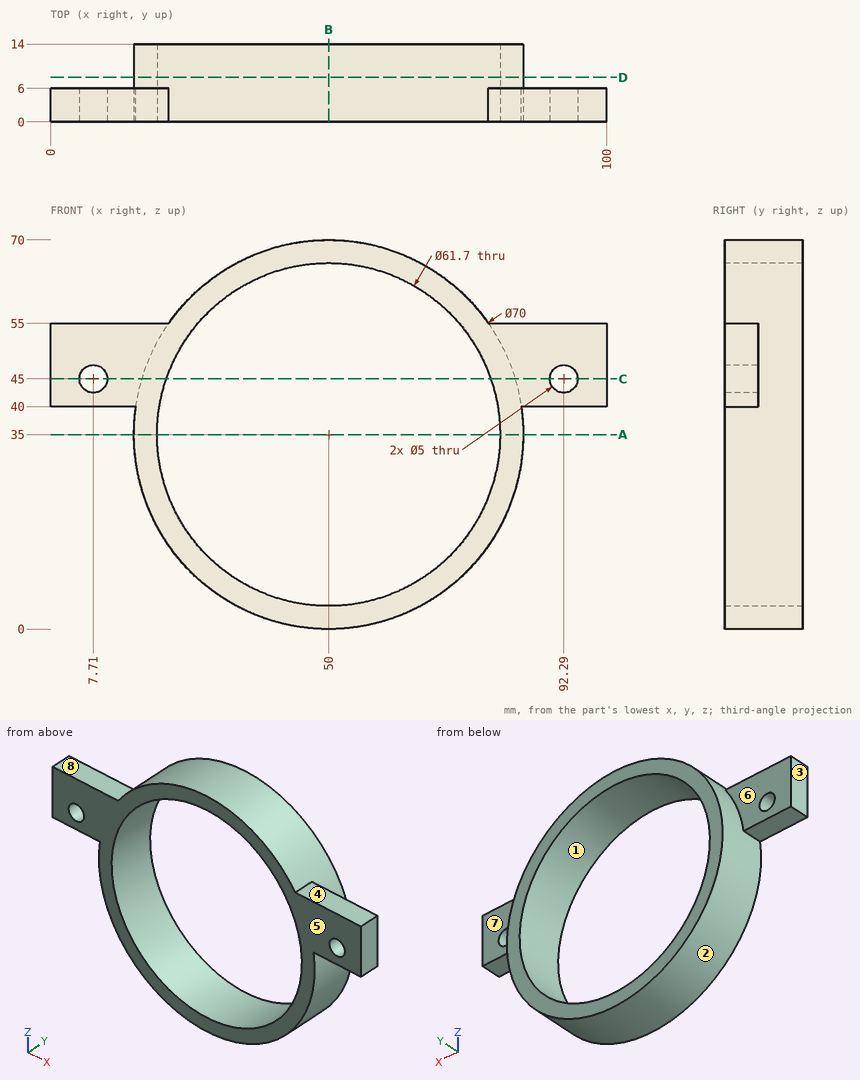
Could you check a few things on this drawing? It's one solid part, dimensions in mm from its lowest x, y, z. A direction names the side the tool comes from. Give positions to 0.01 mm unless a question says otherwise; leave off trailing zeros. Write each loop counter-clockwise with the first axis right and the second up, starting at its lowest first coordinate (ties: lowest second). Pieces come first, ordered by that corner, then holes. Notation, with made-up numbers: (16.25, -33) -> (32.25, -33) arc R20 cw to (32.25, 3) -> close; hole circle Ø2 at (20, -8). An arc over 180 degrees is marked (long way). Answer as a JSON object with one key per item and string values.
Q1. Which directions (+Z, -Z, +X, -X, +Y, -Y) give clear straight access to the entire face, cutting with the end or side of a thin tool? Please do the marked faces 5, 6, 7 and 8.
Taken from the geometry:
{"face 5": "+Z, -Z, +X, -X, -Y", "face 6": "+Z, -X, +Y", "face 7": "+Z, +X, +Y", "face 8": "+Z, -X, +Y, -Y"}
Q2. Suppose I cut it at C-C on z = 45. Write out the boundary of the cut face in (x, y).
Taken from the geometry:
{"outline": "(0, 0) -> (5.21, 0) -> (5.21, 6) -> (0, 6) -> close; (10.21, 0) -> (20.82, 0) -> (20.82, 14) -> (16.46, 14) -> (16.46, 6) -> (10.21, 6) -> close; (79.18, 0) -> (89.79, 0) -> (89.79, 6) -> (83.54, 6) -> (83.54, 14) -> (79.18, 14) -> close; (94.79, 0) -> (100, 0) -> (100, 6) -> (94.79, 6) -> close"}
Q3. Please list where these lines run through material, in increasing order: L1, parallel to X at y = 3, z = 35; L2, parallel to X at y = 2.45, z = 45; L3, parallel to X at y = 10.5, z = 57.
Taken from the geometry:
{"L1": "x = 15 to 19.15, 80.85 to 85", "L2": "x = 0 to 5.21, 10.21 to 20.82, 79.18 to 89.79, 94.79 to 100", "L3": "x = 22.78 to 28.37, 71.63 to 77.22"}
Q4. Suppose I cut it at D-D on y = 8. Write out the boundary of the cut face in (x, z).
Taken from the geometry:
{"outline": "circle Ø70 at (50, 35); hole circle Ø61.7 at (50, 35)"}
Q5. Suppose I cut it at A-A on z = 35. Write out the boundary of the cut face in (x, y), then the cut area to 3 significant figures.
Taken from the geometry:
{"outline": "(15, 0) -> (19.15, 0) -> (19.15, 14) -> (15, 14) -> close; (80.85, 0) -> (85, 0) -> (85, 14) -> (80.85, 14) -> close", "area": "116 mm²"}
Q6. Suppose I cut it at B-B on x = 50. Write out the boundary of the cut face in (y, z), then the cut area to 3 significant figures.
Taken from the geometry:
{"outline": "(0, 0) -> (14, 0) -> (14, 4.15) -> (0, 4.15) -> close; (0, 65.85) -> (14, 65.85) -> (14, 70) -> (0, 70) -> close", "area": "116 mm²"}
Q7. Will these pins go through, and if not, where does the flat tip stop? pin 1 Ø1.5 at (x, y) = (13, 10) entering from -Z; pin 2 Ø6 at (x, y) = (64.5, 3.5) entering from +Z; pin 3 Ø3 at (x, y) = (89, 2) entering from -Z; pin 4 Ø3 at (x, y) = (13, 3) entering from +Z.
Taken from the geometry:
{"pin 1": "passes through", "pin 2": "stops at z = 68.06", "pin 3": "stops at z = 40", "pin 4": "stops at z = 55"}
Q8. We'd pull the mould along X, two halves only. Please class the marked faces 1, 2, 3 and 4: released by +X, released by -X, zero draft, split by the parting line, or undercut.
Taken from the geometry:
{"face 1": "undercut", "face 2": "split by the parting line", "face 3": "released by -X", "face 4": "zero draft"}
